The drawing under review shows one solid part. Ordinate dimensions are in mm from its lowest x, y, z. Give positions to 0.01 mm unless a question says otherwise; leave off trailing zeros. Loops run counter-clockwise (first coordinate to the right, second up) from the corner with the lowest first, then second, coordinate; pieces in that order, holes last.
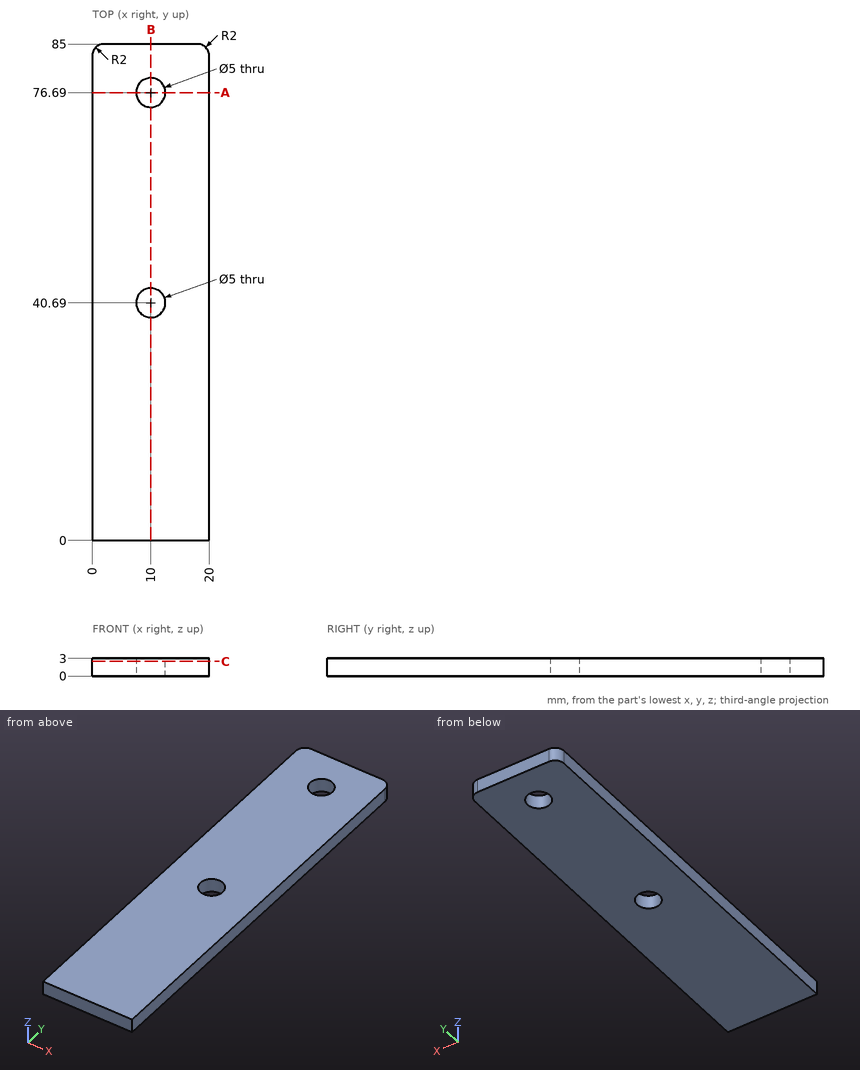
Item 1: Take a section at A-A on y = 76.69. Give the boundary of the cut face in (x, z), and give its area (3 significant figures).
Answer:
outline: (0, 0) - (7.5, 0) - (7.5, 3) - (0, 3) - close; (12.5, 0) - (20, 0) - (20, 3) - (12.5, 3) - close
area: 45.0 mm2
Item 2: Take a section at B-B on x = 10. Give the boundary of the cut face in (y, z), and give its area (3 significant figures).
Answer:
outline: (0, 0) - (38.19, 0) - (38.19, 3) - (0, 3) - close; (43.19, 0) - (74.19, 0) - (74.19, 3) - (43.19, 3) - close; (79.19, 0) - (85, 0) - (85, 3) - (79.19, 3) - close
area: 225 mm2
Item 3: For L1, parallel to Y at x = 10, z = 1.45; L2, parallel to Y at x = 12, z = 2.4; L3, parallel to X at y = 39, z = 1.25, list the stretches that pass through material, from the lowest coordinate up.
Answer:
L1: y = 0 to 38.19, 43.19 to 74.19, 79.19 to 85
L2: y = 0 to 39.19, 42.19 to 75.19, 78.19 to 85
L3: x = 0 to 8.16, 11.84 to 20
Item 4: Clearance check with a flat-ended pin moving along its axis: pin 1 Ø2 at (x, y) = (3, 32.5) entering from -Z. State where the tip first meets the part, or that it passes through.
Answer:
pin 1: stops at z = 0
Item 5: Take a section at C-C on z = 2.5. Give the boundary of the cut face in (x, y).
Answer:
outline: (0, 0) - (20, 0) - (20, 83) arc R2 ccw to (18, 85) - (2, 85) arc R2 ccw to (0, 83) - close; hole circle Ø5 at (10, 40.69); hole circle Ø5 at (10, 76.69)
